For this review, take the finished solid that the model builds, in its own axes (mm). A direction names the side the tool comes from. Coordinates: 2 decimals unless noted, no trailing zeros. Write each loop counter-clockwise with the first axis right and the second up, starting at its lowest first coordinate (ties: lowest second). Pieces come first, ordered by that corner, then holes. Notation, with made-up numbers: (-39, -33) -> (-27, -33) arc R16 cw to (-27, -23) -> close; hole circle Ø6 at (-7.75, -15). An arc over 180 degrees is marked (long way). Put each result on its own line as item: value. Start each with the question number.
Item 1: Consider section D-D on z = 4.75. Give the boundary of the cut face in (x, y), and give its area (3 significant figures).
Item 2: Consider section C-C on x = 7.5. Give the boundary of the cut face in (y, z).
Item 3: Consider section B-B on y = 0. Give the boundary of the cut face in (x, z).
Item 4: The part is to be moulded in two halves that separate along X. For faces 4 (the flat face through (8, -15, 12)), 5 (the flat face through (0, -2, 13)), 6 (the flat face through (24.9, -10.2, 11)), 7 (the cylindrical face through (17.87, 13.19, 7.1)), say which applies: +X half, -X half, draft (parallel to the pull), parting line (faces both ways), or undercut.
Item 5: Insertion check: P1, Ø0.5, axis at x = 23, y = -12.5, coming from the -Z side; P2, Ø3, axis at x = 26.5, y = -2.5, coming from the -Z side. Each pin has a flat end and moves straight along its axis. Give the tip position at first contact, or say it passes through.
Item 6: To check wall thickness, follow L1, parallel to X at y = 12.2, z = 10; L2, parallel to X at y = -9.8, z = 8; L3, parallel to Y at x = 18, z = 10. State the ranges of each line that lie inside material, in increasing order.
Item 7: Consider section A-A on z = 7.75. Give the boundary of the cut face in (x, y), and give its area (3 significant figures).
Item 8: For faces 1 (the flat face through (4, -15, 10)), 2 (the flat face through (25, 14, 9)), 3 (the flat face through (24.9, 10.2, 11)), list the 3-axis set-ups (+Z, -Z, +X, -X, +Y, -Y) from which the entire face can be reached by the end or side of a thin tool; tool diameter is ignored.
```python
from build123d import *

# Parameters (mm, degrees)
EXTRUDE_1_DEPTH     = 20
SKETCH_2_W          = 1
SKETCH_2_H          = 24.4
EXTRUDE_2_DEPTH     = 10
EXTRUDE_4_DEPTH     = 0.6
EXTRUDE_5_DEPTH     = 10
SKETCH_8_W          = 8
SKETCH_8_H          = 4
EXTRUDE_6_DEPTH     = 5.2
EXTRUDE_7_DEPTH     = 3
SKETCH_3_R          = 1
CUT_EXTRUDE_1_DEPTH = 38.682887363
SKETCH_10_W         = 10
SKETCH_10_H         = 9
CUT_EXTRUDE_2_DEPTH = 3


with BuildPart() as part:
    # 草图1 → 凸台-拉伸1 (new body)
    with BuildSketch(Plane(origin=(0, 0, 0), x_dir=(0, 0, -1), z_dir=(1, 0, 0))):
        with BuildLine():
            Line((0, 12.2), (-14, 12.2))
            Line((-14, 12.2), (-14, -12.2))
            Line((-14, -12.2), (0, -12.2))
            ThreePointArc((0, -12.2), (-12.2, 0), (0, 12.2))
        make_face()
    extrude(amount=EXTRUDE_1_DEPTH)

    # 草图2 → 凸台-拉伸2 (add)
    with BuildSketch(Plane(origin=(20, 0, 0), x_dir=(0, 0, -1), z_dir=(1, 0, 0))):
        with Locations((-13.5, 0)):
            Rectangle(SKETCH_2_W, SKETCH_2_H)
    extrude(amount=EXTRUDE_2_DEPTH)

    # 草图6 → 凸台-拉伸4 (add)
    with BuildSketch(Plane.XZ.offset(12.2)):
        Polygon((0, 14), (0, 0), (20, 0), (20, 13), (30, 13), (30, 14), align=None)
    extrude(amount=EXTRUDE_4_DEPTH)

    # 草图7 → 凸台-拉伸5 (add)
    with BuildSketch(Plane(origin=(20, 0, 0), x_dir=(0, 0, -1), z_dir=(1, 0, 0))):
        Polygon((0, -12.2), (-9, -12.2), (-13, -8.2), (-13, -12.8), (0, -12.8), align=None)
        Polygon((-13, 8.2), (-9, 12.2), (-13, 12.2), align=None)
    extrude(amount=EXTRUDE_5_DEPTH)

    # 草图8 → 凸台-拉伸6 (add)
    with BuildSketch(Plane.XZ.offset(12.8)):
        with Locations((4, 12)):
            Rectangle(SKETCH_8_W, SKETCH_8_H)
        with Locations((26, 12)):
            Rectangle(SKETCH_8_W, SKETCH_8_H)
    extrude(amount=EXTRUDE_6_DEPTH)

    # 草图9 → 凸台-拉伸7 (add)
    with BuildSketch(Plane(origin=(0, 12.2, 0), x_dir=(1, 0, 0), z_dir=(0, 1, 0))):
        Polygon((0, 0), (20, 0), (20, -9), (30, -9), (30, -14), (0, -14), align=None)
    extrude(amount=EXTRUDE_7_DEPTH)

    # 草图3 → 切除-拉伸1 (cut, through all)
    with BuildSketch(Plane.XY.offset(14)):
        with Locations((18, 12.2)):
            Circle(SKETCH_3_R)
        with Locations((18, -9.8)):
            Circle(SKETCH_3_R)
    extrude(amount=-CUT_EXTRUDE_1_DEPTH, mode=Mode.SUBTRACT)

    # 草图10 → 切除-拉伸2 (cut)
    with BuildSketch(Plane(origin=(0, -12.2, 0), x_dir=(1, 0, 0), z_dir=(0, 1, 0))):
        with Locations((25, -4.5)):
            Rectangle(SKETCH_10_W, SKETCH_10_H)
    extrude(amount=-CUT_EXTRUDE_2_DEPTH, mode=Mode.SUBTRACT)


solid = part.part
```
Return value:
1. outline: (0, -12.8) -> (20, -12.8) -> (20, -11.24) -> (0, -11.24) -> close; (0, 11.24) -> (17.73, 11.24) arc R1 cw (long way) to (18.27, 11.24) -> (20, 11.24) -> (20, 15.2) -> (0, 15.2) -> close
1. area: 107 mm^2
2. outline: (-18, 10) -> (-12.8, 10) -> (-12.8, 0) -> (-12.2, 0) arc R12.2 cw to (12.2, 0) -> (15.2, 0) -> (15.2, 14) -> (-18, 14) -> close
3. outline: (0, 12.2) -> (20, 12.2) -> (20, 13) -> (30, 13) -> (30, 14) -> (0, 14) -> close
4. face 4: undercut
4. face 5: -X half
4. face 6: draft
4. face 7: undercut
5. P1: z = 9
5. P2: z = 13
6. L1: 0 to 17, 19 to 30
6. L2: 0 to 17, 19 to 20
6. L3: -12.8 to -10.8, -8.8 to -6.99, 6.99 to 11.2, 13.2 to 15.2
7. outline: (0, -12.8) -> (20, -12.8) -> (20, -9.42) -> (18.93, -9.42) arc R1 cw (long way) to (17.07, -9.42) -> (0, -9.42) -> close; (0, 9.42) -> (20, 9.42) -> (20, 15.2) -> (0, 15.2) -> close; hole circle Ø2 at (18, 12.2)
7. area: 178 mm^2
8. face 1: -Z, +X, -X, -Y
8. face 2: -Z, +X, +Y, -Y
8. face 3: -Z, +X
